from build123d import *

# Parameters (mm, degrees)
CROQUIS1_R              = 3.25
SALIENTE_EXTRUIR1_DEPTH = 600


with BuildPart() as part:
    # Croquis1 → Saliente-Extruir1 (new body)
    with BuildSketch(Plane.XY):
        with BuildLine():
            Line((17.638588183, 7.000000593), (15.9, 7.000000593))
            ThreePointArc((15.9, 7.000000593), (15.546446609, 6.853553983), (15.4, 6.500000593))
            Line((15.4, 6.500000593), (15.4, 5.144079725))
            ThreePointArc((15.4, 5.144079725), (15.735093193, 4.335093193), (16.544079725, 4))
            Line((16.544079725, 4), (18.8, 4))
            ThreePointArc((18.8, 4), (19.648528137, 4.351471863), (20, 5.2))
            Line((20, 5.2), (20, 16))
            ThreePointArc((20, 16), (18.828427125, 18.828427125), (16, 20))
            Line((16, 20), (5.2, 20))
            ThreePointArc((5.2, 20), (4.351471862, 19.648528137), (4, 18.8))
            Line((4, 18.8), (4, 16.544079725))
            ThreePointArc((4, 16.544079725), (4.335093193, 15.735093193), (5.144079725, 15.4))
            Line((5.144079725, 15.4), (6.500000593, 15.4))
            ThreePointArc((6.500000593, 15.4), (6.853553983, 15.546446609), (7.000000593, 15.9))
            Line((7.000000593, 15.9), (7.000000593, 17.638588183))
            ThreePointArc((7.000000593, 17.638588183), (7.081377983, 17.823253941), (7.272577483, 17.887802162))
            ThreePointArc((7.272577483, 17.887802162), (9.057180209, 17.101396285), (9.99999956, 15.394254591))
            Line((9.99999956, 15.394254591), (9.99999956, 14.133359942))
            ThreePointArc((9.99999956, 14.133359942), (9.617015406, 12.207968581), (8.52636881, 10.575700602))
            Line((8.52636881, 10.575700602), (6.732513057, 8.781844848))
            ThreePointArc((6.732513057, 8.781844848), (5.47882541, 7.944157544), (4, 7.650000881))
            Line((4, 7.650000881), (-3.999999119, 7.650000881))
            ThreePointArc((-3.999999119, 7.650000881), (-5.478824529, 7.944157544), (-6.732512176, 8.781844848))
            Line((-6.732512176, 8.781844848), (-8.526367489, 10.575700161))
            ThreePointArc((-8.526367489, 10.575700161), (-9.617014085, 12.207968141), (-9.999998238, 14.133359502))
            Line((-9.999998238, 14.133359502), (-9.999998238, 15.394254272))
            ThreePointArc((-9.999998238, 15.394254272), (-9.057177493, 17.101391964), (-7.272576853, 17.887795559))
            ThreePointArc((-7.272576853, 17.887795559), (-7.081377376, 17.823247322), (-7, 17.638581577))
            Line((-7, 17.638581577), (-7, 15.9))
            ThreePointArc((-7, 15.9), (-6.853553391, 15.546446609), (-6.5, 15.4))
            Line((-6.5, 15.4), (-5.144079725, 15.4))
            ThreePointArc((-5.144079725, 15.4), (-4.335093193, 15.735093193), (-4, 16.544079725))
            Line((-4, 16.544079725), (-4, 18.8))
            ThreePointArc((-4, 18.8), (-4.351471863, 19.648528137), (-5.2, 20))
            Line((-5.2, 20), (-16, 20))
            ThreePointArc((-16, 20), (-18.828427125, 18.828427125), (-20, 16))
            Line((-20, 16), (-20, 5.2))
            ThreePointArc((-20, 5.2), (-19.648528137, 4.351471862), (-18.8, 4))
            Line((-18.8, 4), (-16.544079725, 4))
            ThreePointArc((-16.544079725, 4), (-15.735093193, 4.335093193), (-15.4, 5.144079725))
            Line((-15.4, 5.144079725), (-15.4, 6.500000593))
            ThreePointArc((-15.4, 6.500000593), (-15.546446609, 6.853553983), (-15.9, 7.000000593))
            Line((-15.9, 7.000000593), (-17.638588183, 7.000000593))
            ThreePointArc((-17.638588183, 7.000000593), (-17.823253941, 7.081377983), (-17.887802162, 7.272577483))
            ThreePointArc((-17.887802162, 7.272577483), (-17.101396286, 9.057180209), (-15.394254591, 9.99999956))
            Line((-15.394254591, 9.99999956), (-14.133359942, 9.99999956))
            ThreePointArc((-14.133359942, 9.99999956), (-12.207968582, 9.617015406), (-10.575700602, 8.52636881))
            Line((-10.575700602, 8.52636881), (-8.781844848, 6.732513057))
            ThreePointArc((-8.781844848, 6.732513057), (-7.944157544, 5.47882541), (-7.650000881, 4))
            Line((-7.650000881, 4), (-7.650000881, -3.999999119))
            ThreePointArc((-7.650000881, -3.999999119), (-7.944157544, -5.478824529), (-8.781844848, -6.732512176))
            Line((-8.781844848, -6.732512176), (-10.575700161, -8.526367489))
            ThreePointArc((-10.575700161, -8.526367489), (-12.207968141, -9.617014085), (-14.133359502, -9.999998238))
            Line((-14.133359502, -9.999998238), (-15.394254272, -9.999998238))
            ThreePointArc((-15.394254272, -9.999998238), (-17.101391964, -9.057177493), (-17.887795559, -7.272576853))
            ThreePointArc((-17.887795559, -7.272576853), (-17.823247322, -7.081377376), (-17.638581577, -7))
            Line((-17.638581577, -7), (-15.9, -7))
            ThreePointArc((-15.9, -7), (-15.546446609, -6.853553391), (-15.4, -6.5))
            Line((-15.4, -6.5), (-15.4, -5.144079725))
            ThreePointArc((-15.4, -5.144079725), (-15.735093193, -4.335093193), (-16.544079725, -4))
            Line((-16.544079725, -4), (-18.8, -4))
            ThreePointArc((-18.8, -4), (-19.648528137, -4.351471863), (-20, -5.2))
            Line((-20, -5.2), (-20, -16))
            ThreePointArc((-20, -16), (-18.828427125, -18.828427125), (-16, -20))
            Line((-16, -20), (-5.2, -20))
            ThreePointArc((-5.2, -20), (-4.351471863, -19.648528137), (-4, -18.8))
            Line((-4, -18.8), (-4, -16.544079725))
            ThreePointArc((-4, -16.544079725), (-4.335093193, -15.735093193), (-5.144079725, -15.4))
            Line((-5.144079725, -15.4), (-6.5, -15.4))
            ThreePointArc((-6.5, -15.4), (-6.853553391, -15.546446609), (-7, -15.9))
            Line((-7, -15.9), (-7, -17.638581577))
            ThreePointArc((-7, -17.638581577), (-7.081377376, -17.823247322), (-7.272576853, -17.887795559))
            ThreePointArc((-7.272576853, -17.887795559), (-9.057177493, -17.101391964), (-9.999998238, -15.394254272))
            Line((-9.999998238, -15.394254272), (-9.999998238, -14.133359502))
            ThreePointArc((-9.999998238, -14.133359502), (-9.617014085, -12.207968141), (-8.526367489, -10.575700161))
            Line((-8.526367489, -10.575700161), (-6.732512176, -8.781844848))
            ThreePointArc((-6.732512176, -8.781844848), (-5.478824529, -7.944157544), (-3.999999119, -7.650000881))
            Line((-3.999999119, -7.650000881), (4, -7.650000881))
            ThreePointArc((4, -7.650000881), (5.47882541, -7.944157544), (6.732513057, -8.781844848))
            Line((6.732513057, -8.781844848), (8.52636881, -10.575700602))
            ThreePointArc((8.52636881, -10.575700602), (9.617015406, -12.207968582), (9.99999956, -14.133359942))
            Line((9.99999956, -14.133359942), (9.99999956, -15.394254591))
            ThreePointArc((9.99999956, -15.394254591), (9.057180209, -17.101396286), (7.272577483, -17.887802162))
            ThreePointArc((7.272577483, -17.887802162), (7.081377983, -17.823253941), (7.000000593, -17.638588183))
            Line((7.000000593, -17.638588183), (7.000000593, -15.9))
            ThreePointArc((7.000000593, -15.9), (6.853553983, -15.546446609), (6.500000593, -15.4))
            Line((6.500000593, -15.4), (5.144079725, -15.4))
            ThreePointArc((5.144079725, -15.4), (4.335093193, -15.735093193), (4, -16.544079725))
            Line((4, -16.544079725), (4, -18.8))
            ThreePointArc((4, -18.8), (4.351471862, -19.648528137), (5.2, -20))
            Line((5.2, -20), (16, -20))
            ThreePointArc((16, -20), (18.828427125, -18.828427125), (20, -16))
            Line((20, -16), (20, -5.2))
            ThreePointArc((20, -5.2), (19.648528137, -4.351471863), (18.8, -4))
            Line((18.8, -4), (16.544079725, -4))
            ThreePointArc((16.544079725, -4), (15.735093193, -4.335093193), (15.4, -5.144079725))
            Line((15.4, -5.144079725), (15.4, -6.5))
            ThreePointArc((15.4, -6.5), (15.546446609, -6.853553391), (15.9, -7))
            Line((15.9, -7), (17.638581577, -7))
            ThreePointArc((17.638581577, -7), (17.823247322, -7.081377376), (17.887795559, -7.272576853))
            ThreePointArc((17.887795559, -7.272576853), (17.101391964, -9.057177493), (15.394254272, -9.999998238))
            Line((15.394254272, -9.999998238), (14.133359502, -9.999998238))
            ThreePointArc((14.133359502, -9.999998238), (12.207968141, -9.617014085), (10.575700161, -8.526367489))
            Line((10.575700161, -8.526367489), (8.781844848, -6.732512176))
            ThreePointArc((8.781844848, -6.732512176), (7.944157544, -5.478824529), (7.650000881, -3.999999119))
            Line((7.650000881, -3.999999119), (7.650000881, 4))
            ThreePointArc((7.650000881, 4), (7.944157544, 5.47882541), (8.781844848, 6.732513057))
            Line((8.781844848, 6.732513057), (10.575700602, 8.52636881))
            ThreePointArc((10.575700602, 8.52636881), (12.207968581, 9.617015406), (14.133359942, 9.99999956))
            Line((14.133359942, 9.99999956), (15.394254591, 9.99999956))
            ThreePointArc((15.394254591, 9.99999956), (17.101396285, 9.057180209), (17.887802162, 7.272577483))
            ThreePointArc((17.887802162, 7.272577483), (17.823253941, 7.081377983), (17.638588183, 7.000000593))
        make_face()
        Circle(CROQUIS1_R, mode=Mode.SUBTRACT)
        with BuildLine():
            Line((-12, -18), (-16, -18))
            ThreePointArc((-16, -18), (-17.414213562, -17.414213562), (-18, -16))
            Line((-18, -16), (-18, -12))
            Line((-18, -12), (-12, -12))
            Line((-12, -12), (-12, -18))
        make_face(mode=Mode.SUBTRACT)
        with BuildLine():
            Line((18, -16), (18, -12))
            Line((18, -12), (12, -12))
            Line((12, -12), (12, -18))
            Line((12, -18), (16, -18))
            ThreePointArc((16, -18), (17.414213562, -17.414213562), (18, -16))
        make_face(mode=Mode.SUBTRACT)
        with BuildLine():
            Line((16, 18), (12, 18))
            Line((12, 18), (12, 12))
            Line((12, 12), (18, 12))
            Line((18, 12), (18, 16))
            ThreePointArc((18, 16), (17.414213562, 17.414213562), (16, 18))
        make_face(mode=Mode.SUBTRACT)
        with BuildLine():
            Line((-18, 16), (-18, 12))
            Line((-18, 12), (-12, 12))
            Line((-12, 12), (-12, 18))
            Line((-12, 18), (-16, 18))
            ThreePointArc((-16, 18), (-17.414213562, 17.414213562), (-18, 16))
        make_face(mode=Mode.SUBTRACT)
    extrude(amount=SALIENTE_EXTRUIR1_DEPTH)


solid = part.part
The model under review builds one solid part; all positions refer to its coordinate system, in mm. Round coordinates to 2 decimals unless told otherwise and drop trailing zeros. Return JSON: item names as keys, results as strings.
(1) For pin 1 (2.5 mm diameter, centred on y = -18, z = 392, fed in from -X); pin 2 (1.9 mm diameter, centred on y = 16.5, z = 297.5, fed in from -X); pin 3 (1.1 mm diameter, centred on x = -17.5, z = 370.5, fed in from +Y); pin 4 (0.5 mm diameter, centred on y = 17, z = 234.5, fed in from +X), all flat-tipped, find the tip position at first contact; note any pin that passes through.
Solved:
{"pin 1": "x = -19.93", "pin 2": "x = -20", "pin 3": "y = 19.89", "pin 4": "x = 19.93"}
(2) For line 1 (X direction, y = -6.5, z = 108); line 2 (X direction, y = -15, z = 399); line 3 (Y direction, x = 0, z = 323), list the stretches that pass through material, from the lowest coordinate up.
Solved:
{"line 1": "-20 to -15.4, -8.57 to 8.57, 15.4 to 20", "line 2": "-20 to -18, -12 to -10, 10 to 12, 18 to 20", "line 3": "-7.65 to -3.25, 3.25 to 7.65"}
(3) Add section A-A on z = 548. State how many separate pieces and enclosed holes the cut face has, plus the area to 3 significant figures.
Solved:
{"separate pieces": "1", "enclosed holes": "5", "area": "680 mm2"}
